Design review of the part built by this model. Coordinates are the model's own, in mm. A direction names the side the tool comes from. Coordinates: 2 decimals unless noted, no trailing zeros. Write each loop counter-clockwise with the first axis right and the second up, starting at its lowest first coordinate (ties: lowest second). Pieces come first, ordered by that corner, then holes. Notation, with made-up numbers: (29.5, 19) - (73.5, 19) arc R24 cw to (73.5, 29) - close; hole circle Ø5 at (-7, 54.5). An arc over 180 degrees is marked (long way). Answer as a JSON object with one key per item and string values.
```python
from build123d import *

# Parameters (mm, degrees)
SKETCH_2_W      = 20
SKETCH_2_H      = 9
EXTRUDE_1_DEPTH = 11
SKETCH_3_W      = 20
SKETCH_3_H      = 11
EXTRUDE_2_DEPTH = 2


with BuildPart() as part:
    # Sketch 1 → Revolve 1 (revolve)
    with BuildSketch(Plane.XY, mode=Mode.PRIVATE) as revolve_1_sk:
        Polygon((0, 90), (24, 90), (24, 86), (22, 86), (22, 4.4), (17.6, 0), (0, 0), align=None)
    revolve(revolve_1_sk.sketch.rotate(Axis((0, 0, 0), (0, 1, 0)), 270), axis=Axis((0, 0, 0), (0, 1, 0)))

    # Sketch 2 → Extrude 1 (add)
    with BuildSketch(Plane(origin=(0, 0, 0), x_dir=(1, 0, 0), z_dir=(0, 1, 0))):
        Rectangle(SKETCH_2_W, SKETCH_2_H)
    extrude(amount=-EXTRUDE_1_DEPTH)

    # Sketch 3 → Extrude 2 (add)
    with BuildSketch(Plane(origin=(0, 0, 0), x_dir=(1, 0, 0), z_dir=(0, 1, 0))):
        Rectangle(SKETCH_3_W, SKETCH_3_H)
    extrude(amount=-EXTRUDE_2_DEPTH)

    # Sketch 4 → Revolve 2 (revolve)
    with BuildSketch(Plane.XY, mode=Mode.PRIVATE) as revolve_2_sk:
        with BuildLine():
            Line((0, -11), (2.5, -11))
            Line((2.5, -11), (2.5, -13.533333333))
            Line((2.5, -13.533333333), (2.6, -13.533333333))
            ThreePointArc((2.6, -13.533333333), (2.882842712, -13.650490621), (3, -13.933333333))
            ThreePointArc((3, -13.933333333), (2.882842712, -14.216176046), (2.6, -14.333333333))
            Line((2.6, -14.333333333), (2.5, -14.333333333))
            Line((2.5, -14.333333333), (2.5, -14.666666667))
            Line((2.5, -14.666666667), (2.142857143, -14.666666667))
            Line((2.142857143, -14.666666667), (2.142857143, -15))
            Line((2.142857143, -15), (0, -15))
            Line((0, -15), (0, -11))
        make_face()
    revolve(revolve_2_sk.sketch.rotate(Axis((0, -15, 0), (0, 1, 0)), 270), axis=Axis((0, -15, 0), (0, 1, 0)))

    # Sketch 5 → Revolve 3 (revolve)
    with BuildSketch(Plane.XY, mode=Mode.PRIVATE) as revolve_3_sk:
        Polygon((-11, -6.5), (-11, -5.825), (-10.775, -5.6), (9.5, -5.6), (9.5, -4.7), (11.7, -4.7), (12, -5), (12, -6.5), align=None)
    revolve(revolve_3_sk.sketch.rotate(Axis((12, -6.5, 0), (-1, 0, 0)), 270), axis=Axis((12, -6.5, 0), (-1, 0, 0)))


solid = part.part
```
(1) Take a section at A-A, the plane y = 74.5. Write out the cut boundary in (x, z).
Solved:
{"outline": "circle Ø44 at (0, 0)"}
(2) Tool access review of faces 1 (the face through (0, -1, 5.5)), 2 (the face through (0, -6, -4.5)), 3 (the face through (-2.44, -14.5, -0.54)): name each direction out of +Z, -Z, +X, -X, +Y, -Y from which nothing blocks a thin tool from reaching the whole face with its end or side.
Solved:
{"face 1": "+Z, +X, -X, -Y", "face 2": "-Z, +X, -X, -Y", "face 3": "-Y"}
(3) For pin 1 (4 mm diameter, centred on y = 40.5, z = -2, fed in from +X); pin 2 (2 mm diameter, centred on x = -0.5, y = 16, fed in from -Z); pin 3 (3 mm diameter, centred on x = -15.5, y = 29, fed in from -Z), all flat-tipped, find the tip position at first contact; note any pin that passes through.
Solved:
{"pin 1": "stops at x = 22", "pin 2": "stops at z = -22", "pin 3": "stops at z = -16.97"}
(4) To check wall thickness, follow line 1 (Y direction, x = 0.5, z = 4); line 2 (Y direction, x = 19.5, z = -11.5); line 3 (Z direction, x = 2, y = -5.5). State the ranges of each line that lie inside material, in increasing order. Write a range as from..to.
Solved:
{"line 1": "y = -11..90", "line 2": "y = 86..90", "line 3": "z = -4.5..4.5"}
(5) The part is to be moulded in two halves that separate along Y. For faces 4 (the face through (10.862, -8.257, -0.39)), 5 (the face through (0, 90, 0)), 6 (the face through (0, -15, 0)), say which applies: pulls with the +Y half, pulls with the -Y half, needs draft (parallel to the pull), parting line crosses it, or undercut.
Solved:
{"face 4": "undercut", "face 5": "pulls with the +Y half", "face 6": "pulls with the -Y half"}
